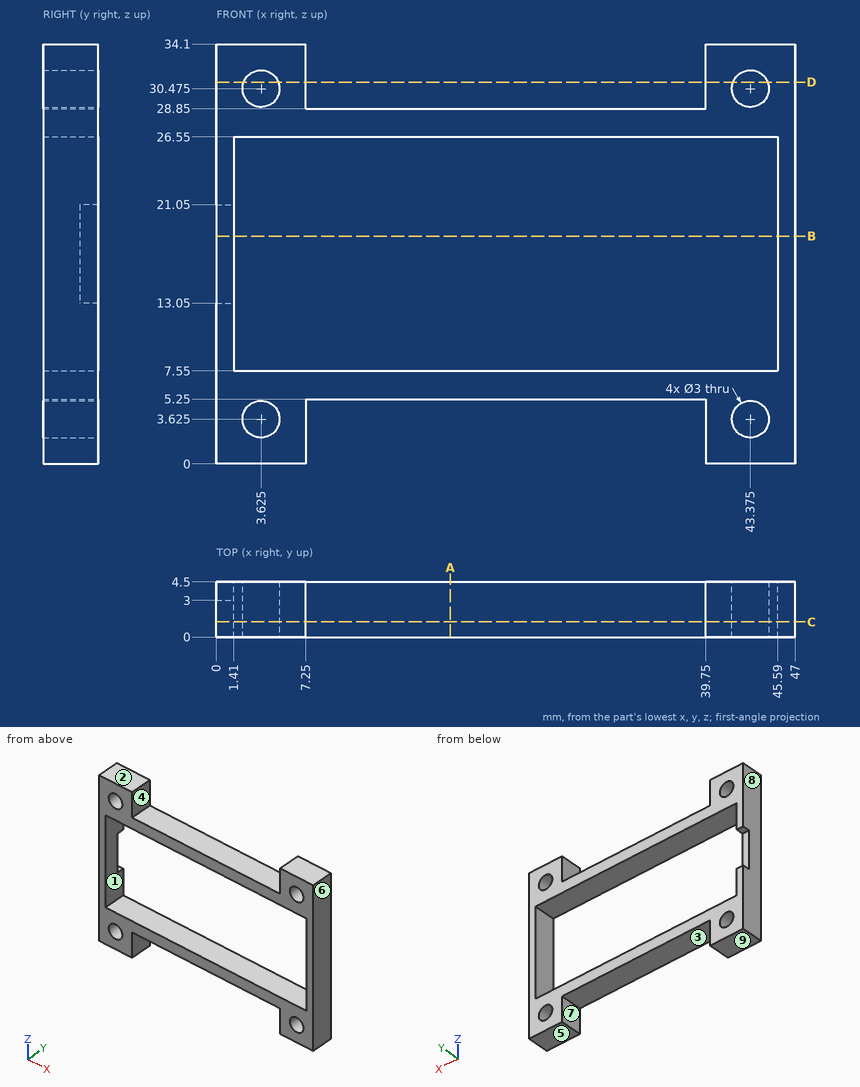
Part print with two shaded views. Sizes in mm from the minimum x, y, z corner. A direction names the side the tool comes from. Round coordinates to 2 decimals unless told otherwise and drop trailing zeros. Loops run counter-clockwise (first coordinate to the right, second up) from the corner with the lowest first, then second, coordinate; pieces in that order, holes last.
Item 1: Saw through at B-B (z = 18.5). List the corners of the cut face in (x, y).
Item 2: Saw through at C-C (y = 1.25). List the corners of the cut face in (x, z) (3 decimals).
Item 3: Saw through at A-A (x = 19). List the corners of the cut face in (y, z), then the cut area to 3 significant figures.
Item 4: Which spindle directions (+Z, -Z, +X, -X, +Y, -Y) get a long thin tool onto all of the face, cutting with end or side? Do the marked faces 1, 2, 3, 4 and 5. Say none if no direction does.
Item 5: Saw through at D-D (z = 31). List the corners of the cut face in (x, y), then the cut area to 3 significant figures.
Item 6: Pin check, flat tips, straight feed: P1, Ø1.3, axis at x = 22, y = 1.5, coming from the -Z side; P2, Ø1.6, axis at x = 1, z = 16, coming from the +Y side; P3, Ø2, axis at x = 29, y = 2, coming from the +Z side. Stop position of each tip, or through.
Item 7: Two-plate mould, pull along X, no slides. Class the marked faces 6, 7, 8 and 9: released by +X, released by -X, zero draft, split by the parting line, or undercut.
Item 8: Drill centre lines: line 1 along Z through (x, y) = (33.5, 2.6); line 2 along Z through (x, y) = (3.5, 0.7); line 3 along X through (y, z) = (1.2, 14). Where is each one in solid material? Low to high.
Worked answers:
1. outline: (0, 0) - (1.41, 0) - (1.41, 3) - (0, 3) - close; (45.59, 0) - (47, 0) - (47, 4.5) - (45.59, 4.5) - close
2. outline: (0, 0) - (7.25, 0) - (7.25, 5.25) - (39.75, 5.25) - (39.75, 0) - (47, 0) - (47, 34.1) - (39.75, 34.1) - (39.75, 28.85) - (7.25, 28.85) - (7.25, 34.1) - (0, 34.1) - close; hole (1.41, 7.55) - (45.59, 7.55) - (45.59, 26.55) - (1.41, 26.55) - close; hole circle Ø3 at (3.625, 3.625); hole circle Ø3 at (3.625, 30.475); hole circle Ø3 at (43.375, 3.625); hole circle Ø3 at (43.375, 30.475)
3. outline: (0, 5.25) - (4.5, 5.25) - (4.5, 7.55) - (0, 7.55) - close; (0, 26.55) - (4.5, 26.55) - (4.5, 28.85) - (0, 28.85) - close
3. area: 20.7 mm2
4. face 1: +Y, -Y
4. face 2: +Z, +X, -X, +Y, -Y
4. face 3: -Z, +Y, -Y
4. face 4: +Z, +Y, -Y
4. face 5: -Z, +X, -X, +Y, -Y
5. outline: (0, 0) - (2.22, 0) - (2.22, 4.5) - (0, 4.5) - close; (5.03, 0) - (7.25, 0) - (7.25, 4.5) - (5.03, 4.5) - close; (39.75, 0) - (41.97, 0) - (41.97, 4.5) - (39.75, 4.5) - close; (44.78, 0) - (47, 0) - (47, 4.5) - (44.78, 4.5) - close
5. area: 40.0 mm2
6. P1: stops at z = 5.25
6. P2: stops at y = 3
6. P3: stops at z = 28.85
7. face 6: released by +X
7. face 7: undercut
7. face 8: released by -X
7. face 9: zero draft
8. line 1: z = 5.25 to 7.55, 26.55 to 28.85
8. line 2: z = 0 to 2.13, 5.12 to 7.55, 26.55 to 28.98, 31.97 to 34.1
8. line 3: x = 0 to 1.41, 45.59 to 47
